Design review of the part shown in the three views and the two pictorial views. Dimensions are in mm from the part's minimum x, y and z. Round coordinates to 2 decimals unless told otherwise and drop trailing zeros. Loops run counter-clockwise (first coordinate to the right, second up) from the corner with the lowest first, then second, coordinate; pieces in that order, holes last.
1) Wall thickness on L1, parallel to Y at x = 4, z = 2; L2, parallel to X at y = 10.75, z = 0.75 (1 decimal); L3, parallel to Y at x = 6.25, z = 6.5 (1 decimal): over which ranges is each line inside the solid? List them lowest first.
2) Insertion check: pin 1 (4.5 mm diameter, centred on x = 4.03, y = 10, fed in from +Z) (3 decimals); pin 2 (6 mm diameter, centred on x = 2.5, y = 11, fed in from +Z); pin 3 (3 mm diameter, centred on y = 10.5, z = 3.5, fed in from +X) (1 decimal). Each pin has a flat end and moves straight along its axis. Give the tip position at first contact, or say it passes through.
3) Mouldability with a two-part tool opening along Y and no side actions: class the marked faces 1, 2, 3 and 4 as pulls with the +Y half, pulls with the -Y half, needs draft (parallel to the pull), parting line crosses it, or undercut.
4) Take a section at C-C (y = 11.5). State the section outline as (x, z) points (1 decimal).
5) Take a section at D-D (x = 8.75). State the section outline as (y, z) points.
6) Take a section at A-A (z = 3.25). State the section outline as (x, y) points (1 decimal).
7) Take a section at B-B (x = 10.25). State the section outline as (y, z) points (1 decimal), then the cut area to 3 significant figures.
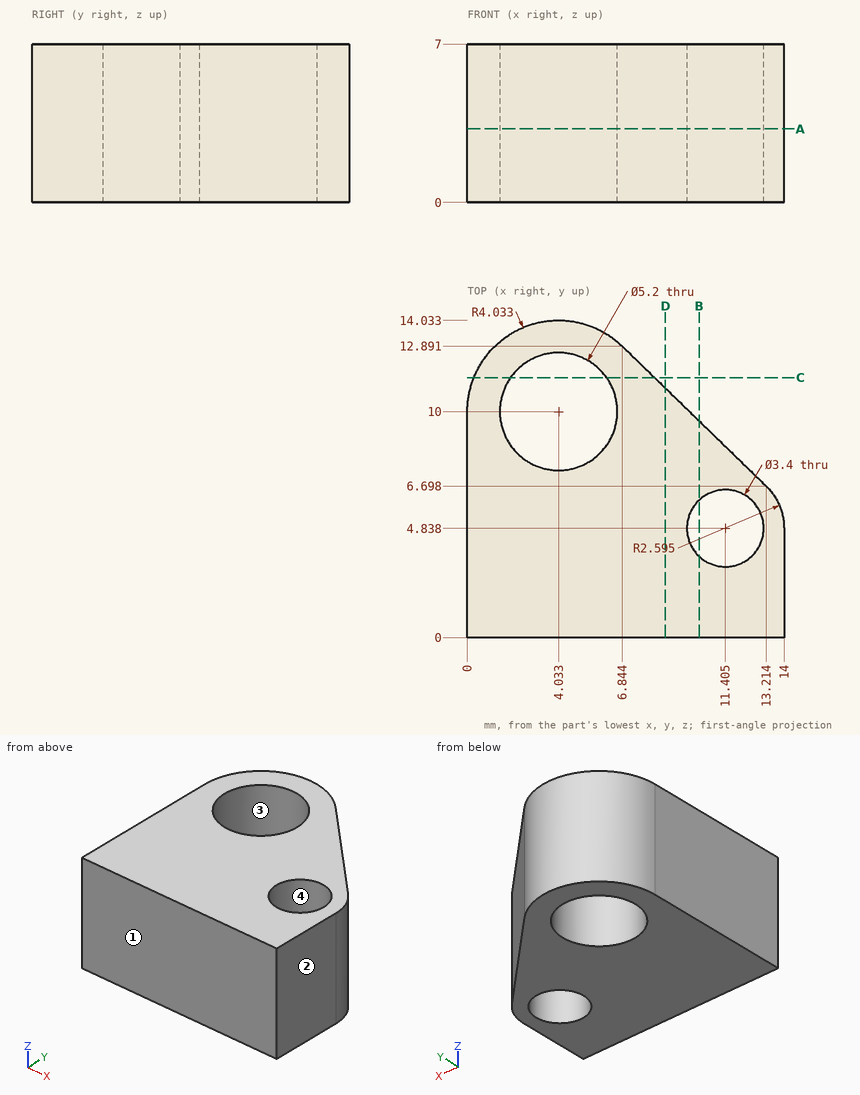
Response:
1. L1: y = 0 to 7.4, 12.6 to 14.03
1. L2: x = 0.1 to 1.5, 6.5 to 9
1. L3: y = 0 to 8.6, 11.4 to 13.4
2. pin 1: passes through
2. pin 2: stops at z = 7
2. pin 3: stops at x = 10.8
3. face 1: pulls with the -Y half
3. face 2: needs draft
3. face 3: undercut
3. face 4: undercut
4. outline: (0.3, 0) - (1.9, 0) - (1.9, 7) - (0.3, 7) - close; (6.2, 0) - (8.3, 0) - (8.3, 7) - (6.2, 7) - close
5. outline: (0, 0) - (11.04, 0) - (11.04, 7) - (0, 7) - close
6. outline: (0, 0) - (14, 0) - (14, 4.8) arc R2.6 ccw to (13.2, 6.7) - (6.8, 12.9) arc R4 ccw to (0, 10) - close; hole circle Ø5.2 at (4, 10); hole circle Ø3.4 at (11.4, 4.8)
7. outline: (0, 0) - (3.6, 0) - (3.6, 7) - (0, 7) - close; (6.1, 0) - (9.6, 0) - (9.6, 7) - (6.1, 7) - close
7. area: 49.6 mm2
